The listing builds one solid part. Answer for the finished solid, in the listing's coordinates (mm). A direction names the side the tool comes from. Give positions to 0.01 mm unless a question says otherwise; leave off trailing zeros. Write each loop counter-clockwise with the first axis right and the second up, starting at its lowest first coordinate (ties: lowest second). Pieces come first, ordered by that corner, then holes. Notation, with made-up numbers: (89, 22) -> (103, 22) arc R22 cw to (103, 49) -> close; hole circle Ø9 at (-15.75, 60.25). An arc over 180 degrees is marked (long way). Put each result on its own line as item: value. Start each with the question number.
1) Find the intervals of material crossed by line 1 along X through (y, z) = (-0.65, 45); line 2 along X through (y, z) = (-0.65, 25); line 3 along X through (y, z) = (-2.1, -21), in increasing order. Write a range as from..to.
2) A cutting plane is placed at D-D (z = -17.5). Write down the section's boundary in (x, y).
3) For faces 1 (the flat face through (1.94, -1, 4)), 2 (the flat face through (26.48, -1.232, 17.504)), determine the directions among +Z, -Z, +X, -X, +Y, -Y from which every point of the face is accessible in a straight line to the end or side of a thin tool.
4) A cutting plane is placed at B-B (x = 9.5). Write down the section's boundary in (y, z), then the cut area to 3 significant figures.
5) A cutting plane is placed at A-A (z = 21). Write down the section's boundary in (x, y), then the cut area to 3 significant figures.
6) Flat-ended cylindrical pins translate along their axes: pin 1 Ø1 at (y, z) = (-0.5, -1.5) entering from -X; pin 2 Ø1.2 at (y, z) = (-1, 46) entering from -X; pin 3 Ø1.5 at (x, y) = (-39, -1) entering from +Z. Find the tip coordinate at first contact, or state that the pin passes through.
7) A cutting plane is placed at C-C (x = 43). Write down the section's boundary in (y, z), then the cut area to 3 significant figures.
8) For a pull along Z with two mould halves and no side action, classify faces 3 (the flat face through (-1, -1, -26.392)), 4 (the flat face through (-1.953, -1, 42)), 5 (the flat face through (0, 0, 8)) as released by +Z, released by -Z, zero draft, split by the parting line, or undercut.
from build123d import *

# Parameters (mm, degrees)
F1_DEPTH = 2.5


with BuildPart() as f1:
    # F0 (on Front) → F1 (new body)
    with BuildSketch(Plane.XZ):
        Polygon((52.2287525237, -26.3921879232), (0, 62.6467168331), (-52.367657423, -26.3921879232), align=None)
        Polygon((25.7395030085, 12.2401500318), (46.4636957768, -23.0901869354), (1.9398448926, -23.0901869354), (-1.9525762507, -23.0901869354), (-46.5948404749, -23.0901869354), (-25.6454423536, 12.5293453449), (-19.8928530583, 22.3102726494), (-1.9525762507, 52.8135007214), (-0.0037810953, 56.1269692776), (1.9398448926, 52.8135007214), (19.728690651, 22.4873055381), align=None, mode=Mode.SUBTRACT)
        with BuildLine():
            ThreePointArc((-1.9525762507, -22.9187820592), (-0.0063822594, -22.989430241), (1.9398448926, -22.9197015464))
            Line((1.9398448926, -22.9197015464), (1.9398448926, -19.7604708833))
            Line((1.9398448926, -19.7604708833), (1.9398448926, -16.0598084555))
            Line((1.9398448926, -16.0598084555), (1.9398448926, -11.5638747518))
            Line((1.9398448926, -11.5638747518), (1.9398448926, -7.9767906652))
            Line((1.9398448926, -7.9767906652), (1.9398448926, -2.8751975899))
            Line((1.9398448926, -2.8751975899), (1.9398448926, 10.9317609152))
            Line((1.9398448926, 10.9317609152), (1.9398448926, 16.0333539904))
            Line((1.9398448926, 16.0333539904), (1.9398448926, 19.620438077))
            Line((1.9398448926, 19.620438077), (1.9398448926, 24.1163717807))
            Line((1.9398448926, 24.1163717807), (1.9398448926, 27.8170342086))
            Line((1.9398448926, 27.8170342086), (1.9398448926, 30.9762648716))
            Line((1.9398448926, 30.9762648716), (1.9398448926, 52.8135007214))
            Line((1.9398448926, 52.8135007214), (-0.0037810953, 56.1269692776))
            Line((-0.0037810953, 56.1269692776), (-1.9525762507, 52.8135007214))
            Line((-1.9525762507, 52.8135007214), (-1.9525762507, 30.9753453844))
            Line((-1.9525762507, 30.9753453844), (-1.9525762507, 27.8159926051))
            Line((-1.9525762507, 27.8159926051), (-1.9525762507, 24.1151382805))
            Line((-1.9525762507, 24.1151382805), (-1.9525762507, 19.6188488698))
            Line((-1.9525762507, 19.6188488698), (-1.9525762507, 16.0312898601))
            Line((-1.9525762507, 16.0312898601), (-1.9525762507, 10.9281707909))
            Line((-1.9525762507, 10.9281707909), (-1.9525762507, -2.8716074657))
            Line((-1.9525762507, -2.8716074657), (-1.9525762507, -7.9747265348))
            Line((-1.9525762507, -7.9747265348), (-1.9525762507, -11.5622855446))
            Line((-1.9525762507, -11.5622855446), (-1.9525762507, -16.0585749552))
            Line((-1.9525762507, -16.0585749552), (-1.9525762507, -19.7594292799))
            Line((-1.9525762507, -19.7594292799), (-1.9525762507, -22.9187820592))
        make_face()
        with BuildLine():
            ThreePointArc((-25.6454423536, 12.5293453449), (-22.4623037962, -10.9851025464), (-1.9525762507, -22.9187820592))
            Line((-1.9525762507, -22.9187820592), (-1.9525762507, -19.7594292799))
            ThreePointArc((-1.9525762507, -19.7594292799), (-23.8677134619, 4.0282816626), (-1.9525762507, 27.8159926051))
            Line((-1.9525762507, 27.8159926051), (-1.9525762507, 30.9753453844))
            ThreePointArc((-1.9525762507, 30.9753453844), (-11.750598572, 28.35687041), (-19.8928530583, 22.3102726494))
            Line((-19.8928530583, 22.3102726494), (-25.6454423536, 12.5293453449))
        make_face()
        with BuildLine():
            Line((1.9398448926, -11.5638747518), (1.9398448926, -16.0598084555))
            ThreePointArc((1.9398448926, -16.0598084555), (20.1815351943, 4.0282816626), (1.9398448926, 24.1163717807))
            Line((1.9398448926, 24.1163717807), (1.9398448926, 19.620438077))
            ThreePointArc((1.9398448926, 19.620438077), (15.712362644, 4.0282816626), (1.9398448926, -11.5638747518))
        make_face()
        with BuildLine():
            ThreePointArc((-1.9525762507, 24.1151382805), (-20.1815351943, 4.0282816626), (-1.9525762507, -16.0585749552))
            Line((-1.9525762507, -16.0585749552), (-1.9525762507, -11.5622855446))
            ThreePointArc((-1.9525762507, -11.5622855446), (-15.712362644, 4.0282816626), (-1.9525762507, 19.6188488698))
            Line((-1.9525762507, 19.6188488698), (-1.9525762507, 24.1151382805))
        make_face()
        with BuildLine():
            ThreePointArc((1.9398448926, -22.9197015464), (22.3738768614, -11.1165666837), (25.7395030085, 12.2401500318))
            Line((25.7395030085, 12.2401500318), (19.728690651, 22.4873055381))
            ThreePointArc((19.728690651, 22.4873055381), (11.636020187, 28.411879253), (1.9398448926, 30.9762648716))
            Line((1.9398448926, 30.9762648716), (1.9398448926, 27.8170342086))
            ThreePointArc((1.9398448926, 27.8170342086), (23.8677134619, 4.0282816626), (1.9398448926, -19.7604708833))
            Line((1.9398448926, -19.7604708833), (1.9398448926, -22.9197015464))
        make_face()
        with BuildLine():
            Line((1.9398448926, -2.8751975899), (1.9398448926, -7.9767906652))
            ThreePointArc((1.9398448926, -7.9767906652), (12.1607877953, 4.0282816626), (1.9398448926, 16.0333539904))
            Line((1.9398448926, 16.0333539904), (1.9398448926, 10.9317609152))
            ThreePointArc((1.9398448926, 10.9317609152), (7.1708454172, 4.0282816626), (1.9398448926, -2.8751975899))
        make_face()
        with BuildLine():
            ThreePointArc((-1.9525762507, 16.0312898601), (-12.1607877953, 4.0282816626), (-1.9525762507, -7.9747265348))
            Line((-1.9525762507, -7.9747265348), (-1.9525762507, -2.8716074657))
            ThreePointArc((-1.9525762507, -2.8716074657), (-7.1708454172, 4.0282816626), (-1.9525762507, 10.9281707909))
            Line((-1.9525762507, 10.9281707909), (-1.9525762507, 16.0312898601))
        make_face()
    extrude(amount=F1_DEPTH)


solid = f1.part
Reply:
1. line 1: x = -10.38..-6.55, -1.95..1.94, 6.52..10.35
1. line 2: x = -22.14..-18.31, -17.03..-11.4, -1.95..1.94, 11.4..17.03, 18.25..22.08
1. line 3: x = -49.2..-45.37, -10.18..10.18, 45.24..49.07
2. outline: (-47.14, -2.5) -> (-43.31, -2.5) -> (-43.31, 0) -> (-47.14, 0) -> close; (-16.32, -2.5) -> (-10.31, -2.5) -> (-10.31, 0) -> (-16.32, 0) -> close; (-1.95, -2.5) -> (1.94, -2.5) -> (1.94, 0) -> (-1.95, 0) -> close; (10.31, -2.5) -> (16.32, -2.5) -> (16.32, 0) -> (10.31, 0) -> close; (43.18, -2.5) -> (47.01, -2.5) -> (47.01, 0) -> (43.18, 0) -> close
3. face 1: +Y, -Y
3. face 2: +Z, +X, +Y, -Y
4. outline: (-2.5, -26.39) -> (0, -26.39) -> (0, -23.09) -> (-2.5, -23.09) -> close; (-2.5, -21.26) -> (0, -21.26) -> (0, -17.87) -> (-2.5, -17.87) -> close; (-2.5, -13.78) -> (0, -13.78) -> (0, -8.49) -> (-2.5, -8.49) -> close; (-2.5, -3.56) -> (0, -3.56) -> (0, 11.62) -> (-2.5, 11.62) -> close; (-2.5, 16.54) -> (0, 16.54) -> (0, 21.83) -> (-2.5, 21.83) -> close; (-2.5, 25.92) -> (0, 25.92) -> (0, 29.32) -> (-2.5, 29.32) -> close; (-2.5, 39.93) -> (0, 39.93) -> (0, 46.45) -> (-2.5, 46.45) -> close
4. area: 106 mm2
5. outline: (-24.49, -2.5) -> (-16.78, -2.5) -> (-16.78, 0) -> (-24.49, 0) -> close; (-10.92, -2.5) -> (10.92, -2.5) -> (10.92, 0) -> (-10.92, 0) -> close; (16.78, -2.5) -> (24.43, -2.5) -> (24.43, 0) -> (16.78, 0) -> close
5. area: 93.0 mm2
6. pin 1: stops at x = -38.02
6. pin 2: stops at x = -10.14
6. pin 3: stops at z = -2.39
7. outline: (-2.5, -26.39) -> (0, -26.39) -> (0, -23.09) -> (-2.5, -23.09) -> close; (-2.5, -17.19) -> (0, -17.19) -> (0, -10.66) -> (-2.5, -10.66) -> close
7. area: 24.6 mm2
8. face 3: released by -Z
8. face 4: undercut
8. face 5: zero draft
